from build123d import *

# Parameters (mm, degrees)
SKETCH1_W                           = 50
SKETCH1_H                           = 40
EXTRUDE1_DEPTH                      = 11.9888
M5X0_8_TAPPED_HOLE1_D               = 4.2
M5X0_8_TAPPED_HOLE1_DEPTH           = 9.5758
M5X0_8_TAPPED_HOLE1_TIP             = 1.2618073
F_1_8_0_125_DIAMETER_HOLE1_D        = 3.175
F_1_8_0_125_DIAMETER_HOLE1_DEPTH    = 6.35
CIRPATTERN1_COUNT                   = 3
F_5_32_0_15625_DIAMETER_HOLE1_D     = 3.96875
F_5_32_0_15625_DIAMETER_HOLE1_DEPTH = 6.2484
M3X0_5_TAPPED_HOLE2_D               = 2.5
M3X0_5_TAPPED_HOLE2_DEPTH           = 5.7912
M3X0_5_TAPPED_HOLE2_TIP             = 0.751075774
CHAMFER1_SIZE                       = 0.762
EXTRUDE2_DEPTH                      = 1.016


with BuildPart() as part:
    # Sketch1 → Extrude1 (new body)
    with BuildSketch(Plane(origin=(0, 0, 0), x_dir=(1, 0, 0), z_dir=(0, 1, 0))):
        Rectangle(SKETCH1_W, SKETCH1_H)
    extrude(amount=EXTRUDE1_DEPTH)

    # M5x0.8 Tapped Hole1
    with Locations(Plane(origin=(0, 0, -20), x_dir=(-1, 0, 0), z_dir=(0, 0, -1))):
        with Locations((0, 5.334)):
            Hole(M5X0_8_TAPPED_HOLE1_D / 2, depth=M5X0_8_TAPPED_HOLE1_DEPTH)
            with Locations((0, 0, -(M5X0_8_TAPPED_HOLE1_DEPTH + M5X0_8_TAPPED_HOLE1_TIP / 2))):  # 118° drill point
                Cone(0, M5X0_8_TAPPED_HOLE1_D / 2, M5X0_8_TAPPED_HOLE1_TIP, mode=Mode.SUBTRACT)

    # 1_8 _0.125_ Diameter Hole1
    with Locations(Plane.XZ):
        with Locations((17, 0)):
            Hole(F_1_8_0_125_DIAMETER_HOLE1_D / 2, depth=F_1_8_0_125_DIAMETER_HOLE1_DEPTH)

    # Sketch8 → M3x0.5 Tapped Hole1 (revolve, cut)
    with BuildSketch(Plane(origin=(-10.795, 0, 0), x_dir=(0, 0, -1), z_dir=(1, 0, 0))):
        Polygon((0, 0), (0, 7.304275774), (1.25, 6.5532), (1.25, 0), align=None)
    m3x0_5_tapped_hole1 = revolve(axis=Axis((-10.795, -6.35, 0), (0, 1, 0)), mode=Mode.SUBTRACT)

    # CirPattern1: M3x0.5 Tapped Hole1 ×3 about axis
    cirpattern1_axis = Axis((0, 0, 0), (0, 1, 0))
    for i in range(1, CIRPATTERN1_COUNT):
        add(m3x0_5_tapped_hole1.rotate(cirpattern1_axis, i * 360 / CIRPATTERN1_COUNT), mode=Mode.SUBTRACT)

    # 5_32 _0.15625_ Diameter Hole1
    with Locations(Plane.XZ):
        with Locations((0, 0)):
            Hole(F_5_32_0_15625_DIAMETER_HOLE1_D / 2, depth=F_5_32_0_15625_DIAMETER_HOLE1_DEPTH)

    # Sketch12 → Cut-Revolve1 (revolve, cut)
    with BuildSketch(Plane.XZ.offset(0.508)):
        with BuildLine():
            Line((0, 6.5024), (0, -6.5024))
            ThreePointArc((0, -6.5024), (6.5024, 0), (0, 6.5024))
        make_face()
    revolve(axis=Axis((0, -0.508, 6.5024), (0, 0, -1)), mode=Mode.SUBTRACT)

    # M3x0.5 Tapped Hole2
    with Locations(Plane.XZ):
        with Locations((-17, 0)):
            Hole(M3X0_5_TAPPED_HOLE2_D / 2, depth=M3X0_5_TAPPED_HOLE2_DEPTH)
            with Locations((0, 0, -(M3X0_5_TAPPED_HOLE2_DEPTH + M3X0_5_TAPPED_HOLE2_TIP / 2))):  # 118° drill point
                Cone(0, M3X0_5_TAPPED_HOLE2_D / 2, M3X0_5_TAPPED_HOLE2_TIP, mode=Mode.SUBTRACT)

    # Chamfer1
    chamfer1_edges = [part.edges().sort_by_distance(p)[0] for p in [
        (0, 0, -20),
        (25, 0, 0),
        (0, 0, 20),
        (-25, 0, 0),
    ]]
    chamfer(chamfer1_edges, length=CHAMFER1_SIZE)

    # Sketch2 → Extrude2 (add)
    with BuildSketch(Plane(origin=(0, 11.9888, 0), x_dir=(-1, 0, 0), z_dir=(0, 1, 0))):
        with BuildLine():
            Line((20.8725, 19.0475), (-20.8851, 19.0475))
            ThreePointArc((-20.8851, 19.0475), (-23.13016403, 18.11756403), (-24.0601, 15.8725))
            Line((-24.0601, 15.8725), (-24.0601, -15.8775))
            ThreePointArc((-24.0601, -15.8775), (-23.13016403, -18.12256403), (-20.8851, -19.0525))
            Line((-20.8851, -19.0525), (20.8725, -19.0525))
            ThreePointArc((20.8725, -19.0525), (23.11756403, -18.12256403), (24.0475, -15.8775))
            Line((24.0475, -15.8775), (24.0475, 15.8725))
            ThreePointArc((24.0475, 15.8725), (23.11756403, 18.11756403), (20.8725, 19.0475))
        make_face()
    extrude(amount=EXTRUDE2_DEPTH)


solid = part.part
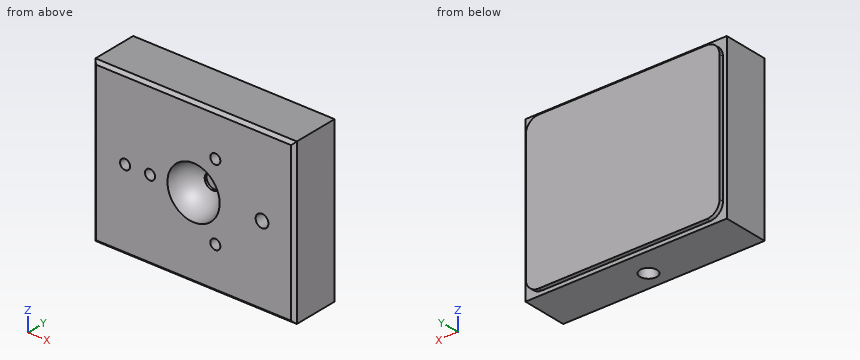
The listing builds one solid part. Answer for the finished solid, in the listing's coordinates (mm). Round coordinates to 2 decimals unless told otherwise and drop trailing zeros. Order: outer loops, then holes, each group sorted by start corner. A loop starts at its lowest first (then second) coordinate and runs counter-clockwise, first axis right, second up. Notation, with made-up numbers: (79, -11) -> (117, -11) arc R14 ccw to (117, 12) -> close; hole circle Ø3 at (3, 72). An arc over 180 degrees is marked (long way). Write each question's results on one line, items separated by ' | '. Start each with the question number.
Q1. Find section A-A (x = 17). Determine the outline of the cut face in (y, z), then the cut area to 3 significant figures.
Q2. Find section B-B (z = -14.5). Determine the outline of the cut face in (x, y), then the cut area to 3 significant figures.
Q3. Each of these flat-tipped pins is pushed along its axis until it touches: pin 1 (0.5 mm diameter, centred on y = 12.5, z = 0, fed in from -X); pin 2 (2.5 mm diameter, centred on x = 0, z = 0, fed in from -Y); pin 3 (4 mm diameter, centred on x = 0, y = 5.334, fed in from -Z). Where does it stop, or does it pass through?
Q4. Straight lines are drawn through the part: probe 1 along X at (y, z) = (6, 0.5); probe 2 along Z at (x, y) = (17, 4); probe 3 along Z at (x, y) = (6.5, 3.75). For each, find the intervals that lie inside material, in ascending order. Write a range as from..to.
Worked answers:
1) outline: (0, -19.24) -> (0.76, -20) -> (11.99, -20) -> (11.99, -19.05) -> (13, -19.05) -> (13, 19.05) -> (11.99, 19.05) -> (11.99, 20) -> (0.76, 20) -> (0, 19.24) -> (0, 1.59) -> (6.35, 1.59) -> (6.35, -1.59) -> (0, -1.59) -> close | area: 498 mm2
2) outline: (-25, 0.76) -> (-24.24, 0) -> (24.24, 0) -> (25, 0.76) -> (25, 11.99) -> (24.06, 11.99) -> (24.06, 13) -> (-24.05, 13) -> (-24.05, 11.99) -> (-25, 11.99) -> close; hole circle Ø4.2 at (0, 5.33) | area: 634 mm2
3) pin 1: stops at x = -24.05 | pin 2: stops at y = 6.25 | pin 3: stops at z = -10.36
4) probe 1: x = -25..-17.75, -16.25..-11.94, -9.65..-1.92, 1.92..15.49, 18.51..25 | probe 2: z = -20..-1.59, 1.59..20 | probe 3: z = -20..-9.94, -8.76..8.76, 9.94..20
